```python
from build123d import *

# Parameters (mm, degrees)
EXTRUDE003_DEPTH  = 3.6
CYLINDER002_R     = 1.35
CYLINDER002_DEPTH = 3.4
EXTRUDE002_DEPTH  = 1.8
CYLINDER003_R     = 1.35
CYLINDER003_DEPTH = 3.4
EXTRUDE001_DEPTH  = 1.8
CYLINDER_R        = 1.35
CYLINDER_DEPTH    = 3.4
BOX_W             = 22
BOX_H             = 3.4
BOX_DEPTH         = 14.5
BOX001_W          = 12.7
BOX001_H          = 4.6
BOX001_DEPTH      = 3.4
EXTRUDE_DEPTH     = 3.4


with BuildPart() as extrude003:
    # Sketch003 → Extrude003 (new body)
    with BuildSketch(Plane(origin=(16.5, -1, 1.6), x_dir=(1, 0, 0), z_dir=(0, 0, 1))):
        Polygon((2.8868, 0), (1.4434, 2.500042), (-1.4434, 2.500042), (-2.8868, 0), (-1.4434, -2.500042), (1.4434, -2.500042), align=None)
    extrude(amount=EXTRUDE003_DEPTH)


with BuildPart() as hole03:
    # Cylinder002 → Cylinder002 (new body)
    with BuildSketch(Plane(origin=(16.5, -1, 0), x_dir=(0, 1, 0), z_dir=(0, 0, 1))):
        Circle(CYLINDER002_R)
    extrude(amount=CYLINDER002_DEPTH)

    # Fusion002: union Extrude003
    add(extrude003.part)


with BuildPart() as extrude002:
    # Sketch002 → Extrude002 (new body)
    with BuildSketch(Plane(origin=(16.5, 1.8, 9), x_dir=(1, 0, 0), z_dir=(0, -1, 0))):
        Polygon((2.8868, 0), (1.4434, 2.500042), (-1.4434, 2.500042), (-2.8868, 0), (-1.4434, -2.500042), (1.4434, -2.500042), align=None)
    extrude(amount=EXTRUDE002_DEPTH)


with BuildPart() as hole02:
    # Cylinder003 → Cylinder003 (new body)
    with BuildSketch(Plane(origin=(16.5, 3.4, 9), x_dir=(1, 0, 0), z_dir=(0, -1, 0))):
        Circle(CYLINDER003_R)
    extrude(amount=CYLINDER003_DEPTH)

    # Fusion001: union Extrude002
    add(extrude002.part)


with BuildPart() as extrude001:
    # Sketch001 → Extrude001 (new body)
    with BuildSketch(Plane(origin=(5.5, 1.8, 9), x_dir=(1, 0, 0), z_dir=(0, -1, 0))):
        Polygon((2.8868, 0), (1.4434, 2.500042), (-1.4434, 2.500042), (-2.8868, 0), (-1.4434, -2.500042), (1.4434, -2.500042), align=None)
    extrude(amount=EXTRUDE001_DEPTH)


with BuildPart() as hole01:
    # Cylinder → Cylinder (new body)
    with BuildSketch(Plane(origin=(5.5, 3.4, 9), x_dir=(1, 0, 0), z_dir=(0, -1, 0))):
        Circle(CYLINDER_R)
    extrude(amount=CYLINDER_DEPTH)

    # Fusion: union Extrude001
    add(extrude001.part)


with BuildPart() as cut001:
    # Box → Box (new body)
    with BuildSketch(Plane.XY):
        with Locations((11, 1.7)):
            Rectangle(BOX_W, BOX_H)
    extrude(amount=BOX_DEPTH)

    # Cut: cut Hole01
    add(hole01.part, mode=Mode.SUBTRACT)

    # Cut001: cut Hole02
    add(hole02.part, mode=Mode.SUBTRACT)


with BuildPart() as cut002:
    # Box001 → Box001 (new body)
    with BuildSketch(Plane(origin=(9.3, -4.6, 0), x_dir=(1, 0, 0), z_dir=(0, 0, 1))):
        with Locations((6.35, 2.3)):
            Rectangle(BOX001_W, BOX001_H)
    extrude(amount=BOX001_DEPTH)

    # Fusion003: union Cut001
    add(cut001.part)

    # Cut002: cut Hole03
    add(hole03.part, mode=Mode.SUBTRACT)


with BuildPart() as right_hand_bracket:
    # Sketch → Extrude (new body)
    with BuildSketch(Plane(origin=(0, 0, 3.4), x_dir=(0, 1, 0), z_dir=(1, 0, 0))):
        Polygon((0, 11.1), (0, 0), (-4.6, 0), align=None)
    extrude(amount=EXTRUDE_DEPTH)


with BuildPart() as right_hand_bracket_1:
    # Extrude placement: moved
    add(right_hand_bracket.part.moved(Location((9.3, 0, 0))))

    # Fusion004: union Cut002
    add(cut002.part)


solid = right_hand_bracket_1.part
```
Part model, mm, in its own coordinate system. A direction names the side the tool comes from. Give positions to 0.01 mm unless a question says otherwise; leave off trailing zeros. Order: outer loops, then holes, each group sorted by start corner. A loop starts at its lowest first (then second) coordinate and runs counter-clockwise, first axis right, second up. Notation, with made-up numbers: M -10,67 L 20,67 A29 ccw 20,102 Z; hole C 8.25,16 d8. An arc over 180 degrees is marked long. Use a Markdown table: item, result. Add a question column.
(1) Probe line 1 along X through (y, z) = (2.85, 9); line 2 along X through (y, z) = (-1, 0.8); line 3 along Z through (x, y) = (16.5, 2.6). List the from-to ranges inside material, lowest first. Write a range as [from, to].
(2) 3-axis set-ups, long thin cutter, end or side, ignore diameter. For faces 4 (the face through (18.655, 0.913, 7.732)), 5 (the face through (14.51, 0.55, 2.97)), 6 (the face through (18.655, -2.268, 2.487)): which of +Z, -Z, +X, -X, +Y, -Y reach the whole face in a straight line?
(3) Saw through at C-C, the plane x = 16.5. Give the cut face in (y, z), and give its area (3 significant figures).
(4) Drop flat-ended pins along their axis: P1, Ø4, axis at x = 18.5, z = 12.5, coming from the -Y side; P2, Ø3.5, axis at x = 19, y = -2, coming from the +Z side; P3, Ø1.5, axis at x = 17, y = -1.5, coming from the +Z side; P4, Ø1.6, axis at x = 5.5, z = 9, coming from the -Y side. Give the stop position or say it passes through.
(5) Saw through at D-D, the plane y = 2.5. Give the cut face in (x, z).
(6) Saw through at A-A, the plane x = 5.5. Give the cut face in (y, z), and give its area (3 significant figures).
(7) Saw through at B-B, the plane y = 1. Give the cut face in (x, z).
(8) Mould opens along Z. For faces 1 (the face through (10.976, -2.332, 8.872)), 2 (the face through (3.325, 0.913, 7.767)), 3 (the face through (0, 2, 7)) say: +Z half, -Z half, draft (parallel to the pull), parting line (faces both ways), or undercut.
Answer key:
| question | item | result |
|---|---|---|
| 1 | line 1 | [0, 4.15], [6.85, 15.15], [17.85, 22] |
| 1 | line 2 | [9.3, 15.15], [17.85, 22] |
| 1 | line 3 | [0, 7.65], [10.35, 14.5] |
| 2 | face 4 | -Y |
| 2 | face 5 | none |
| 2 | face 6 | +Z |
| 3 | outline | M -4.6,0 L -2.35,0 L -2.35,1.6 L -3.5,1.6 L -3.5,3.4 L -4.6,3.4 Z; M 0,5.2 L 1.5,5.2 L 1.5,1.6 L 0.35,1.6 L 0.35,0 L 3.4,0 L 3.4,7.65 L 1.8,7.65 L 1.8,6.5 L 0,6.5 Z; M 0,11.5 L 1.8,11.5 L 1.8,10.35 L 3.4,10.35 L 3.4,14.5 L 0,14.5 Z |
| 3 | area | 35.6 mm^2 |
| 4 | P1 | y = 0 |
| 4 | P2 | z = 3.4 |
| 4 | P3 | z = 1.6 |
| 4 | P4 | through |
| 5 | outline | M 0,0 L 22,0 L 22,14.5 L 0,14.5 Z; hole C 5.5,9 d2.7; hole C 16.5,9 d2.7 |
| 6 | outline | M 0,0 L 3.4,0 L 3.4,7.65 L 1.8,7.65 L 1.8,6.5 L 0,6.5 Z; M 0,11.5 L 1.8,11.5 L 1.8,10.35 L 3.4,10.35 L 3.4,14.5 L 0,14.5 Z |
| 6 | area | 36.0 mm^2 |
| 7 | outline | M 0,0 L 22,0 L 22,14.5 L 0,14.5 Z; hole M 2.61,9 L 4.06,6.5 L 6.94,6.5 L 8.39,9 L 6.94,11.5 L 4.06,11.5 Z; hole M 13.61,9 L 15.06,6.5 L 17.94,6.5 L 19.39,9 L 17.94,11.5 L 15.06,11.5 Z; hole M 14.77,1.6 L 18.23,1.6 L 18.23,5.2 L 14.77,5.2 Z |
| 8 | face 1 | +Z half |
| 8 | face 2 | undercut |
| 8 | face 3 | draft |
